Can you work these out from the drawing? Everything is in mm from the part's minimum corner. A direction names the side the tool comes from. Round coordinates to 2 decimals unless told otherwise and drop trailing zeros. Loops run counter-clockwise (first coordinate to the right, second up) from the corner with the lowest first, then second, coordinate; pieces in that order, holes last. Notation, with made-up numbers: (-35.5, 26.25) -> (-29.5, 26.25) arc R25 ccw to (-29.5, 40.25) -> close; hole circle Ø7 at (79, 58). An arc over 180 degrees is marked (long way). One line per item, written item: value.
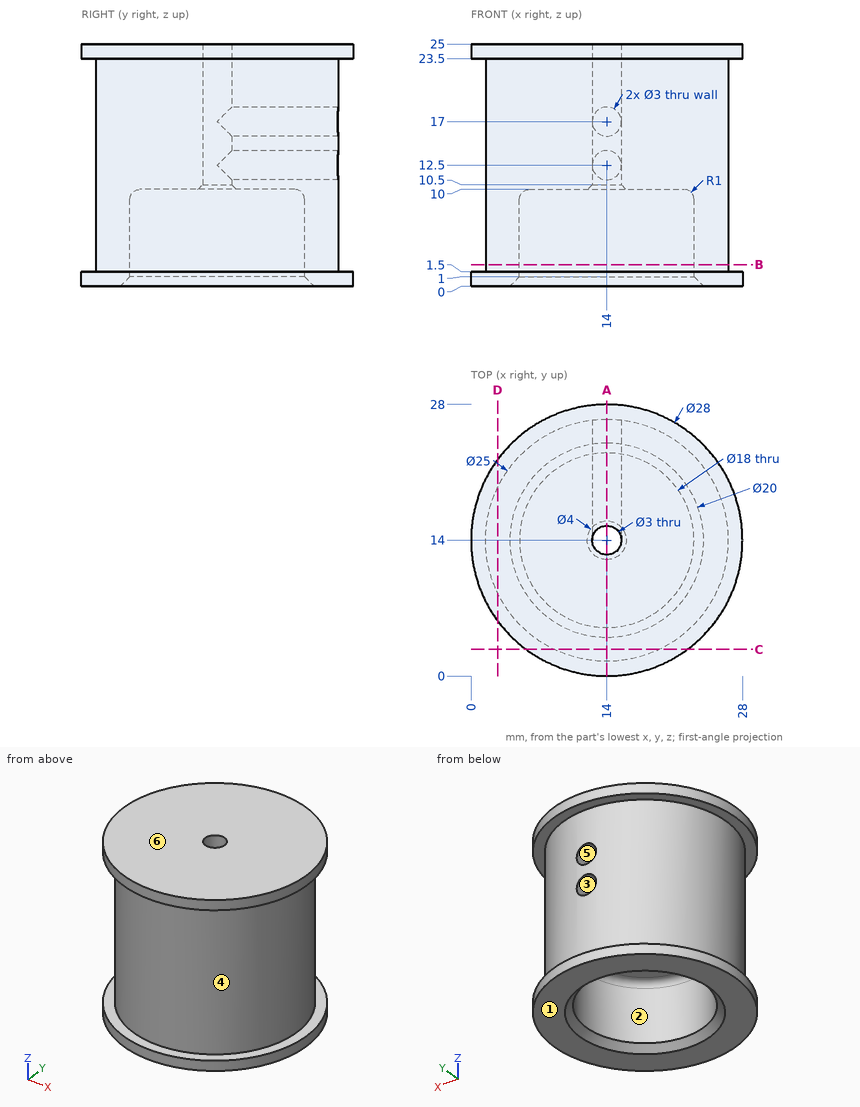
(1) If we section it at A-A, the plane x = 14: Give the number of separate pieces and of enclosed holes in the cut face, then the cut area to 3 significant figures.
Recorded:
separate pieces: 4
enclosed holes: 0
area: 342 mm²
(2) I'm going to push flat-ended pins straight in: pin 1 Ø8 at (x, y) = (12, 13.5) entering from -Z; pin 2 Ø4 at (x, z) = (14, 12.5) entering from +Y; pin 3 Ø2 at (x, z) = (21, 20) entering from -Y; pin 4 Ø12 at (x, z) = (13, 21) entering from -Y. Where does each tip first touch, or does it pass through?
Recorded:
pin 1: z = 10
pin 2: y = 26.5
pin 3: y = 3.03
pin 4: y = 0
(3) If we section it at C-C, the plane y = 2.75: Please give me the cut outline in (x, z), then the cut area to 3 significant figures.
Recorded:
outline: (5.67, 0) -> (22.33, 0) -> (22.33, 1.5) -> (19.45, 1.5) -> (19.45, 23.5) -> (22.33, 23.5) -> (22.33, 25) -> (5.67, 25) -> (5.67, 23.5) -> (8.55, 23.5) -> (8.55, 1.5) -> (5.67, 1.5) -> close
area: 290 mm²
(4) Thinking about a two-plate mould opening in X: for the marked faces 3, 4, 5 and 6, which applies, released by +X, released by -X, zero draft, split by the parting line, or undercut?
Recorded:
face 3: undercut
face 4: split by the parting line
face 5: undercut
face 6: zero draft
(5) If we section it at B-B, the plane z = 2.25: Please give me the cut outline in (x, y).
Recorded:
outline: circle Ø25 at (14, 14); hole circle Ø18 at (14, 14)
(6) If I drill on L1, parallel to Z at x = 14, y = 17.5; L2, parallel to Z at x = 5.75, y = 24.75; L3, parallel to Z at x = 14.5, y = 10.5, over which ranges is the centre line in solid material (lowest first)?
Recorded:
L1: 10 to 11, 14 to 15.5, 18.5 to 25
L2: 0 to 1.5, 23.5 to 25
L3: 10 to 25
(7) For the marked faces 1 and 2, which set-ups out of +Z, -Z, +X, -X, +Y, -Y let a thin tool reach every point of the face, with its end or its side?
Recorded:
face 1: -Z, +X, -X, +Y, -Y
face 2: -Z
